The model under review builds one solid part; all positions refer to its coordinate system, in mm. A direction names the side the tool comes from. Coordinates: 2 decimals unless noted, no trailing zeros. Write each loop counter-clockwise with the first axis right and the second up, starting at its lowest first coordinate (ties: lowest second). Pieces come first, ordered by that corner, then holes.
Autodesk Inventor part; units mm, degrees
ref_plane "YZ Plane" through (0, 0, 0) normal (1, 0, 0) x (0, 1, 0)
ref_plane "XZ Plane" through (0, 0, 0) normal (0, 1, 0) x (-1, 0, 0)
ref_plane "XY Plane" through (0, 0, 0) normal (0, 0, 1) x (1, 0, 0)
sketch "スケッチ1" plane through (0, 0, 0) normal (1, 0, 0) x (0, 1, 0)
  point P0 (0, 0)
sketch "スケッチ2" plane through (0, 0, 0) normal (0, 0, 1) x (1, 0, 0)
  line L0 (-3.75, 7.5) -> (3.75, 7.5)
  line L1 (3.75, 7.5) -> (3.75, -7.5)
  line L2 (3.75, -7.5) -> (-3.75, -7.5)
  line L3 (-3.75, -7.5) -> (-3.75, 7.5)
  line L4 (-3.75, 7.5) -> (3.75, -7.5) construction
  line L5 (3.75, 7.5) -> (-3.75, -7.5) construction
  point P0 (0, 0)
  dimension "d0" = 7.5
  dimension "d1" = 15
extrude "押し出し1" add sketch "スケッチ2" along normal blind 12
sketch "スケッチ3" plane through (-3.75, 7.5, 0) normal (0, 1, 0) x (1, 0, 0)
  circle A0 centre (3.75, -9.5) radius 1.25
  point P0 (3.75, 0)
  dimension "d4" = 2.5
extrude "押し出し2" cut sketch "スケッチ3" against normal blind 6
sketch "スケッチ4" plane through (3.75, -7.5, 0) normal (1, 0, 0) x (0, 0, -1)
  circle A0 centre (-8.3, 7.5) radius 1.5
  point P0 (0, 7.5)
  dimension "d7" = 3
extrude "押し出し3" cut sketch "スケッチ4" against normal blind 20
sketch "スケッチ5" plane through (3.75, -7.5, 0) normal (1, 0, 0) x (0, 0, -1)
  circle A0 centre (-4.25, 2.5) radius 1.5
  circle A1 centre (-4.25, 12.5) radius 1.5
  point P0 (0, 7.5)
  dimension "d10" = 3
  dimension "d11" = 3
extrude "押し出し4" cut sketch "スケッチ5" against normal blind 20
sketch "スケッチ6" plane through (3.75, -7.5, 0) normal (1, 0, 0) x (0, 0, -1)
  circle A0 centre (-4.25, 2.5) radius 1.5
  circle A1 centre (-4.25, 2.5) radius 3.5
  circle A2 centre (-4.25, 12.5) radius 1.5
  circle A3 centre (-4.25, 12.5) radius 3.5
  point P0 (0, 7.5)
  dimension "d14" = 7
  dimension "d15" = 7
extrude "押し出し5" add sketch "スケッチ6" against normal blind 10
sketch "スケッチ7" plane through (-3.75, -7.5, 12) normal (0, -1, 0) x (1, 0, 0)
  arc A0 (4.1, -3.7) -> (3.4, -3.7) centre (3.75, -2.5) ccw
  circle A1 centre (3.75, -2.5) radius 1.25
  point P0 (3.75, -12)
extrude "押し出し6" cut sketch "スケッチ7" against normal blind 6
thread "ねじ1"
thread "ねじ2"
properties part number "moving_part" material "アルミニウム"
Item 1: Take a section at B-B, the plane y = 2.5. Write out the cut boundary in (x, z), plus the area to 3 significant figures.
Solved:
outline: (-6.25, 1.8) - (-3.75, 1.8) - (-3.75, 0) - (3.75, 0) - (3.75, 12) - (-3.75, 12) - (-3.75, 6.7) - (-6.25, 6.7) - close; hole circle Ø2.5 at (0, 9.5)
area: 97.3 mm2
Item 2: For pin 1 (3 mm diameter, centred on x = 0, z = 9.5, fed in from -Y); pin 2 (2 mm diameter, centred on x = -0.5, z = 6, fed in from +Y); pin 3 (2 mm diameter, centred on x = 0, z = 9, fed in from +Y); pin 4 (1.8 mm diameter, centred on y = 5, z = 4.25, fed in from -X), all flat-tipped, find the tip position at first contact; note any pin that passes through.
Solved:
pin 1: stops at y = -7.5
pin 2: stops at y = 8.42
pin 3: stops at y = 7.5
pin 4: passes through
Item 3: Take a section at A-A, the plane y = -6.25. Write out the cut boundary in (x, z).
Solved:
outline: (-6.25, 0.98) - (-3.75, 0.98) - (-3.75, 0) - (3.75, 0) - (3.75, 3.42) - (-6.25, 3.42) - close; (-6.25, 5.08) - (3.75, 5.08) - (3.75, 12) - (-3.75, 12) - (-3.75, 7.52) - (-6.25, 7.52) - close; hole circle Ø2.5 at (0, 9.5)
Item 4: To check wall thickness, follow line 1 along Z through (x, y) = (0, 5.1); line 2 along Y through (x, z) = (-1.75, 4.25); line 3 along Y through (x, z) = (1, 8.3). State the ranges of each line that lie inside material, in increasing order.
Solved:
line 1: z = 0 to 2.75, 5.75 to 8.25, 10.75 to 12
line 2: y = -8.5 to -6.5, -3.5 to 3.5, 6.5 to 8.5
line 3: y = -7.5 to -1.5, 1.5 to 7.5
Item 5: Take a section at D-D, the plane x = -2.75. Write out the cut boundary in (y, z).
Solved:
outline: (-7.5, 0) - (7.5, 0) - (7.5, 1.8) arc R3.5 ccw to (7.5, 6.7) - (7.5, 12) - (-7.5, 12) - (-7.5, 6.7) arc R3.5 ccw to (-7.5, 1.8) - close; hole circle Ø3 at (-5, 4.25); hole circle Ø3 at (0, 8.3); hole circle Ø3 at (5, 4.25)
Item 6: Machinability: for faces 1 (the face through (0, 7.5, 8)), 2 (the face through (-3.402, -8.417, 5.009)), 3 (the face through (-0.136, -4.542, 8.257)), 4 (the face through (0, -7.5, 1)), which of the approach directions +Z, -Z, +X, -X, +Y, -Y give a long, thin tool a straight path to every point of the face, cutting with its end or side? Answer none if there is none.
Solved:
face 1: +Z, +X, -X, +Y
face 2: -X
face 3: -Y
face 4: -Z, +X, -X, -Y
Item 7: Take a section at C-C, the plane z = 4.25. Write out the cut boundary in (x, y), plus the area to 4 significant figures.
Solved:
outline: (-6.25, -8.5) - (3.75, -8.5) - (3.75, -6.5) - (-6.25, -6.5) - close; (-6.25, -3.5) - (3.75, -3.5) - (3.75, 3.5) - (-6.25, 3.5) - (-6.25, 1.5) - (-3.75, 1.5) - (-3.75, -1.5) - (-6.25, -1.5) - close; (-6.25, 6.5) - (3.75, 6.5) - (3.75, 8.5) - (-6.25, 8.5) - close
area: 102.5 mm2
Item 8: Mouldability with a two-part tool opening along X and no side actions: class faces 5 (the face through (3.75, 0, 6)), 6 (the face through (0.672, 4.542, 8.446)), 7 (the face through (0, 0, 0)) as pulls with the +X half, pulls with the -X half, needs draft (parallel to the pull), parting line crosses it, or undercut.
Solved:
face 5: pulls with the +X half
face 6: undercut
face 7: needs draft
